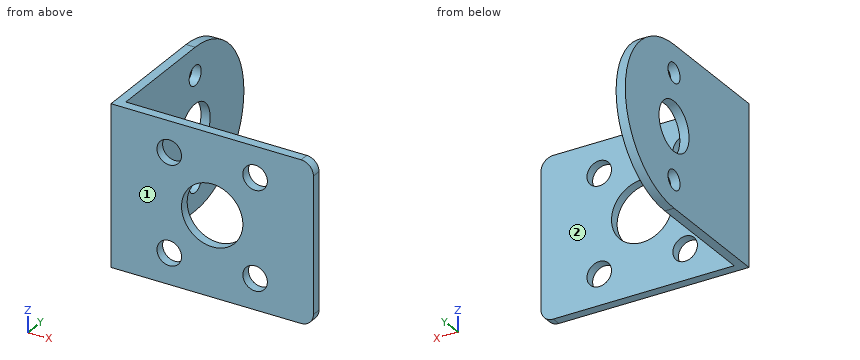
from build123d import *

# Parameters (mm, degrees)
BOSS_EXTRUDE1_DEPTH = 26
FILLET1_R           = 2
SKETCH3_R           = 5
SKETCH3_R_2         = 2
CUT_EXTRUDE1_DEPTH  = 53.509522946
SKETCH4_R           = 4
SKETCH4_R_2         = 1.6
CUT_EXTRUDE2_DEPTH  = 53.509522946


with BuildPart() as part:
    # Sketch2 → Boss-Extrude1 (new body)
    with BuildSketch(Plane.XY):
        Polygon((0, 0), (33, 0), (33, 1.5), (1.5, 1.5), (1.5, 33), (0, 33), align=None)
    extrude(amount=BOSS_EXTRUDE1_DEPTH)

    # Fillet1
    fillet1_edges = [part.edges().sort_by_distance(p)[0] for p in [
        (33, 0.75, 26),
        (33, 0.75, 0),
    ]]
    fillet(fillet1_edges, radius=FILLET1_R)

    # Sketch3 → Cut-Extrude1 (cut, through all)
    with BuildSketch(Plane(origin=(0, 1.5, 0), x_dir=(1, 0, 0), z_dir=(0, 1, 0))):
        with Locations(Location((16.5, -13, 0), (0, 0, 180))):
            Circle(SKETCH3_R)
        with Locations(Location((9.5, -5, 0), (0, 0, 180))):
            Circle(SKETCH3_R_2)
        with Locations(Location((23.5, -5, 0), (0, 0, 180))):
            Circle(SKETCH3_R_2)
        with Locations(Location((23.5, -21, 0), (0, 0, 180))):
            Circle(SKETCH3_R_2)
        with Locations(Location((9.5, -21, 0), (0, 0, 180))):
            Circle(SKETCH3_R_2)
    extrude(amount=-CUT_EXTRUDE1_DEPTH, mode=Mode.SUBTRACT)

    # Sketch4 → Cut-Extrude2 (cut, through all)
    with BuildSketch(Plane(origin=(1.5, 0, 0), x_dir=(0, 0, -1), z_dir=(1, 0, 0))):
        with Locations(Location((-13, 20, 0), (0, 0, 90))):
            Circle(SKETCH4_R)
        with Locations(Location((-21.5, 20, 0), (0, 0, 90))):
            Circle(SKETCH4_R_2)
        with Locations(Location((-4.5, 20, 0), (0, 0, 90))):
            Circle(SKETCH4_R_2)
        with BuildLine():
            Line((-26, 20), (-26, 38.59710215))
            Line((-26, 38.59710215), (0, 38.59710215))
            Line((0, 38.59710215), (0, 20))
            ThreePointArc((0, 20), (-13, 33), (-26, 20))
        make_face()
    extrude(amount=-CUT_EXTRUDE2_DEPTH, mode=Mode.SUBTRACT)


solid = part.part
Source: CAD feature listing. Evaluate the final solid. Frame: model axes, mm. Face numbers are marked on the shaded views. A direction names the side the tool comes from. Round coordinates to 2 decimals unless told otherwise and drop trailing zeros. Loops run counter-clockwise (first coordinate to the right, second up) from the corner with the lowest first, then second, coordinate; pieces in that order, holes last. Notation, with made-up numbers: M 15.5,-6.5 L 44.5,-6.5 A27 cw 44.5,30.5 Z; hole C 30,9.25 d9. An arc over 180 degrees is marked long. Return JSON: item names as keys, results as strings. Group by question number.
1. Section query C-C on y = 17. Output: boundary loops of the cut face in (x, z).
2. Section query B-B on z = 13. Output: boundary loops of the cut face in (x, y), and give its area (4 significant figures).
3. Material intervals for line 1 along Z through (x, y) = (1, 20); line 2 along Z through (x, y) = (23.5, 1.25); line 3 along Z through (x, y) = (16.5, 0.75), sorted ascending. Write a range as from..to.
4. Section query D-D on x = 16.5. Output: boundary loops of the cut face in (y, z), and give its area (3 significant figures).
5. Pin query (flat end, axial travel): pin 1 (4.5 mm diameter, centred on x = 23.5, z = 21, fed in from +Y); pin 2 (3 mm diameter, centred on y = 20, z = 4.5, fed in from -X); pin 3 (13 mm diameter, centred on y = 16, z = 17.5, fed in from +X); pin 4 (12 mm diameter, centred on y = 14.5, z = 5, fed in from -X). Return the tip coordinate at first contact, or that it passes through.
6. Section query A-A on x = 23.5. Output: boundary loops of the cut face in (y, z), and give its area (3 significant figures).
7. Reachability of the marked faces 1 and 2 from +Z, -Z, +X, -X, +Y, -Y: full face, straight path, thin tool, end or side. Return the list, or none.
Checks:
{
 "1": {"outline": "M 0,0 L 1.5,0 L 1.5,10.35 L 0,10.35 Z; M 0,15.65 L 1.5,15.65 L 1.5,26 L 0,26 Z"},
 "2": {"outline": "M 0,0 L 11.5,0 L 11.5,1.5 L 1.5,1.5 L 1.5,16 L 0,16 Z; M 0,24 L 1.5,24 L 1.5,33 L 0,33 Z; M 21.5,0 L 33,0 L 33,1.5 L 21.5,1.5 Z", "area": "69.75 mm²"},
 "3": {"line 1": "z = 0..2.9, 6.1..9, 17..19.9, 23.1..26", "line 2": "z = 0..3, 7..19, 23..26", "line 3": "z = 0..8, 18..26"},
 "4": {"outline": "M 0,0 L 1.5,0 L 1.5,8 L 0,8 Z; M 0,18 L 1.5,18 L 1.5,26 L 0,26 Z", "area": "24.0 mm²"},
 "5": {"pin 1": "stops at y = 1.5", "pin 2": "passes through", "pin 3": "stops at x = 1.5", "pin 4": "stops at x = 0"},
 "6": {"outline": "M 0,0 L 1.5,0 L 1.5,3 L 0,3 Z; M 0,7 L 1.5,7 L 1.5,19 L 0,19 Z; M 0,23 L 1.5,23 L 1.5,26 L 0,26 Z", "area": "27.0 mm²"},
 "7": {"face 1": "+Z, -Z, +X, -X, -Y", "face 2": "+Z, -Z, +X, +Y"}
}
